from build123d import *

# Parameters (mm, degrees)
ESBO_O1_W                = 40
ESBO_O1_H                = 96
ESBO_O1_W_2              = 34.5
ESBO_O1_H_2              = 90.5
RESSALTO_EXTRUS_O1_DEPTH = 10
ESBO_O2_W                = 40
ESBO_O2_H                = 96
RESSALTO_EXTRUS_O2_DEPTH = 3
ESBO_O3_R                = 3.5
CORTE_EXTRUS_O1_DEPTH    = 3
ESBO_O4_W                = 12
ESBO_O4_H                = 10
CORTE_EXTRUS_O2_DEPTH    = 3
FILETE1_R                = 3
ESBO_O5_RX               = 3.5
ESBO_O5_RY               = 3.5
ESBO_O5_W                = 12
ESBO_O5_H                = 10
RESSALTO_EXTRUS_O3_DEPTH = 3
ESBO_O6_R                = 3.5
CORTE_EXTRUS_O3_DEPTH    = 3
ESBO_O7_W                = 12
ESBO_O7_H                = 10
CORTE_EXTRUS_O4_DEPTH    = 3
ESBO_O8_R                = 3.5
ESBO_O8_W                = 12
ESBO_O8_H                = 10
RESSALTO_EXTRUS_O4_DEPTH = 3
ESBO_O9_R                = 3.5
ESBO_O9_W                = 12
ESBO_O9_H                = 10
CORTE_EXTRUS_O5_DEPTH    = 3


with BuildPart() as part:
    # Esboço1 → Ressalto-extrusão1 (new body)
    with BuildSketch(Plane(origin=(0, 0, 0), x_dir=(1, 0, 0), z_dir=(0, 1, 0))):
        with Locations((-1.557629238, 0.07005309)):
            Rectangle(ESBO_O1_W, ESBO_O1_H)
        with Locations((-1.307629238, -0.17994691)):
            Rectangle(ESBO_O1_W_2, ESBO_O1_H_2, mode=Mode.SUBTRACT)
    extrude(amount=RESSALTO_EXTRUS_O1_DEPTH)

    # Esboço2 → Ressalto-extrusão2 (add)
    with BuildSketch(Plane(origin=(0, 10, 0), x_dir=(1, 0, 0), z_dir=(0, 1, 0))):
        with Locations((-1.557629238, 0.07005309)):
            Rectangle(ESBO_O2_W, ESBO_O2_H)
    extrude(amount=RESSALTO_EXTRUS_O2_DEPTH)

    # Esboço3 → Corte-extrusão1 (cut)
    with BuildSketch(Plane.XZ.offset(-10)):
        with Locations(Location((-4.557629238, 23.42994691, 0), (0, 0, 270))):
            Circle(ESBO_O3_R)
    extrude(amount=-CORTE_EXTRUS_O1_DEPTH, mode=Mode.SUBTRACT)

    # Esboço4 → Corte-extrusão2 (cut)
    with BuildSketch(Plane.XZ.offset(-10)):
        with Locations((-7.557629238, -36.07005309)):
            Rectangle(ESBO_O4_W, ESBO_O4_H)
    extrude(amount=-CORTE_EXTRUS_O2_DEPTH, mode=Mode.SUBTRACT)

    # Filete1
    filete1_edges = [part.edges().sort_by_distance(p)[0] for p in [
        (-21.557629238, 13, -0.07005309),
        (-1.557629238, 13, 47.92994691),
        (18.442370762, 13, -0.07005309),
        (-1.557629238, 13, -48.07005309),
        (-21.557629238, 6.5, -48.07005309),
        (18.442370762, 6.5, -48.07005309),
        (18.442370762, 6.5, 47.92994691),
        (-21.557629238, 6.5, 47.92994691),
    ]]
    fillet(filete1_edges, radius=FILETE1_R)

    # Esboço5 → Ressalto-extrusão3 (add)
    with BuildSketch(Plane.XZ.offset(-10)):
        with Locations(Location((-4.557629238, 23.42994691), (0, 0, -90))):
            Ellipse(ESBO_O5_RX, ESBO_O5_RY)
        with Locations((-7.557629238, -36.07005309)):
            Rectangle(ESBO_O5_W, ESBO_O5_H)
    extrude(amount=-RESSALTO_EXTRUS_O3_DEPTH)

    # Esboço6 → Corte-extrusão3 (cut)
    with BuildSketch(Plane.XZ.offset(-10)):
        with Locations(Location((-2.557629238, 20.92994691, 0), (0, 0, 270))):
            Circle(ESBO_O6_R)
    extrude(amount=-CORTE_EXTRUS_O3_DEPTH, mode=Mode.SUBTRACT)

    # Esboço7 → Corte-extrusão4 (cut)
    with BuildSketch(Plane.XZ.offset(-10)):
        with Locations((-7.557629238, -36.07005309)):
            Rectangle(ESBO_O7_W, ESBO_O7_H)
    extrude(amount=-CORTE_EXTRUS_O4_DEPTH, mode=Mode.SUBTRACT)

    # Esboço8 → Ressalto-extrusão4 (add)
    with BuildSketch(Plane.XZ.offset(-10)):
        with Locations((-2.557629238, 20.92994691)):
            Circle(ESBO_O8_R)
        with Locations((-7.557629238, -36.07005309)):
            Rectangle(ESBO_O8_W, ESBO_O8_H)
    extrude(amount=-RESSALTO_EXTRUS_O4_DEPTH)

    # Esboço9 → Corte-extrusão5 (cut)
    with BuildSketch(Plane(origin=(0, 10, 0), x_dir=(-1, 0, 0), z_dir=(0, -1, 0))):
        with Locations(Location((3.057629238, 20.07005309, 0), (0, 0, 90))):
            Circle(ESBO_O9_R)
        with Locations((-2.442370762, -32.92994691)):
            Rectangle(ESBO_O9_W, ESBO_O9_H)
    extrude(amount=-CORTE_EXTRUS_O5_DEPTH, mode=Mode.SUBTRACT)


solid = part.part
Design review of the part built by this model. Coordinates are the model's own, in mm. A direction names the side the tool comes from. Give positions to 0.01 mm unless a question says otherwise; leave off trailing zeros. Order: outer loops, then holes, each group sorted by start corner. A loop starts at its lowest first (then second) coordinate and runs counter-clockwise, first axis right, second up. Notation, with made-up numbers: (-28, 22) - (26, 22) arc R34 cw to (26, 52) - close; hole circle Ø2 at (52, 64). An arc over 180 degrees is marked (long way). Write item = value, one per line. Start each with the question number.
Q1. We need section A-A on y = 4.5. State the section outline as (x, z) points.
Q2. To check wall thickness, follow L1, parallel to Z at x = -11, y = 1; L2, parallel to X at y = 8.5, z = 5; L3, parallel to Y at x = 6, z = -3. State the ranges of each line that lie inside material, in increasing order. Write a range as from..to.
Q3. We need section B-B on x = -1. State the section outline as (y, z) points.
Q4. We need section D-D on x = -16.5. State the section outline as (y, z) points, plus the area to 3 significant figures.
Q5. Mouldability with a two-part tool opening along Z and no side actions: class faces 1 (the face through (-2, 5, -48.07)), 2 (the face through (-2, 5, 45.43)), 3 (the face through (-2, 5, 47.93)) as released by +Z, released by -Z, zero draft, split by the parting line, or undercut.
Q6. Clearance check with flat-ended pins moving along their axes: pin 1 Ø1.5 at (x, y) = (5, 12) entering from -Z; pin 2 Ø17 at (x, z) = (-5, 10.5) entering from -Y; pin 3 Ø5 at (x, z) = (14.5, -29.5) entering from -Y; pin 4 Ø1.5 at (y, z) = (11.5, 33.5) entering from -X. State where each tip first meets the part, or that it passes through.
Q7. We need section C-C on z = 7.5. State the section outline as (x, y) points.
Q8. Tool access review of faces 4 (the face through (-20.7, 4.93, -47.17)), 5 (the face through (-2, 5, -45.07)), 6 (the face through (3, 11, 27.93)): name each direction out of +Z, -Z, +X, -X, +Y, -Y from which nothing blocks a thin tool from reaching the whole face with its end or side.
Working result:
q1.outline = (-21.56, -45.07) arc R3 ccw to (-18.56, -48.07) - (15.44, -48.07) arc R3 ccw to (18.44, -45.07) - (18.44, 44.93) arc R3 ccw to (15.44, 47.93) - (-18.56, 47.93) arc R3 ccw to (-21.56, 44.93) - close; hole (-18.56, -45.07) - (15.94, -45.07) - (15.94, 45.43) - (-18.56, 45.43) - close
q2.L1 = -48.07..-45.07, 45.43..47.93
q2.L2 = -21.56..-18.56, 15.94..18.44
q2.L3 = 10..13
q3.outline = (0, -48.07) - (10, -48.07) arc R3 ccw to (13, -45.07) - (13, -22.9) - (10, -22.9) - (10, -45.07) - (0, -45.07) - close; (0, 45.43) - (10, 45.43) - (10, 37.93) - (13, 37.93) - (13, 44.93) arc R3 ccw to (10, 47.93) - (0, 47.93) - close; (10, -17.24) - (13, -17.24) - (13, 27.93) - (10, 27.93) - close
q4.outline = (0, -48.07) - (10, -48.07) arc R3 ccw to (13, -45.07) - (13, 44.93) arc R3 ccw to (10, 47.93) - (0, 47.93) - (0, 45.43) - (10, 45.43) - (10, -45.07) - (0, -45.07) - close
q4.area = 339 mm²
q5.face_1 = released by -Z
q5.face_2 = undercut
q5.face_3 = released by +Z
q6.pin_1 = -47.8
q6.pin_2 = 10
q6.pin_3 = 0
q6.pin_4 = -21.46
q7.outline = (-21.56, 0) - (-18.56, 0) - (-18.56, 10) - (15.94, 10) - (15.94, 0) - (18.44, 0) - (18.44, 10) arc R3 ccw to (15.44, 13) - (-18.56, 13) arc R3 ccw to (-21.56, 10) - close
q8.face_4 = -Z, -X, +Y, -Y
q8.face_5 = -Y
q8.face_6 = +Y, -Y
